from build123d import *

# Parameters (mm, degrees)
BOSS_EXTRUDE1_DEPTH = 25


with BuildPart() as part:
    # Sketch1 → Revolve1 (revolve)
    with BuildSketch(Plane(origin=(0, 0, 0), x_dir=(1, 0, 0), z_dir=(0, 1, 0))):
        Polygon((-85, 0), (-85, 100), (-30, 100), (-30, 433.75), (-65, 433.75), (-65, 478.75), (-45, 478.75), (-17.679491924, 471.429491924), (0, 453.75), (0, 0), align=None)
    revolve(axis=Axis((0, 0, 0), (-1, 0, 0)))

    # Sketch2 → Boss-Extrude1 (add)
    with BuildSketch(Plane.ZY.offset(30)):
        with BuildLine():
            Line((20, 105.830052443), (20, 422.686719096))
            ThreePointArc((20, 422.686719096), (23.183829742, 430.003810253), (30.707964602, 432.661626921))
            ThreePointArc((30.707964602, 432.661626921), (-31.38909354, 432.612745197), (-92.842809365, 423.697150391))
            ThreePointArc((-92.842809365, 423.697150391), (-42.387293117, 411.834770603), (-20, 365.087746302))
            Line((-20, 365.087746302), (-20, 105.830052443))
            ThreePointArc((-20, 105.830052443), (-22.022759648, 99.799825551), (-27.272727273, 96.209138584))
            ThreePointArc((-27.272727273, 96.209138584), (0, 100), (27.272727273, 96.209138584))
            ThreePointArc((27.272727273, 96.209138584), (22.022759648, 99.799825551), (20, 105.830052443))
        make_face()
        with BuildLine():
            Line((83.347135305, 68.214771395), (287.018674676, 310.94106015))
            ThreePointArc((287.018674676, 310.94106015), (294.160965293, 314.499750862), (301.633198614, 311.699335889))
            ThreePointArc((301.633198614, 311.699335889), (254.032671724, 351.577109888), (201.225560333, 384.24905513))
            ThreePointArc((201.225560333, 384.24905513), (232.25173743, 342.729764327), (219.352990909, 292.529191499))
            Line((219.352990909, 292.529191499), (52.70535758, 93.926275782))
            ThreePointArc((52.70535758, 93.926275782), (47.279678663, 90.60705882), (40.949921045, 91.231047163))
            ThreePointArc((40.949921045, 91.231047163), (64.278760969, 76.604444312), (82.734163396, 56.169904816))
            ThreePointArc((82.734163396, 56.169904816), (81.020503963, 62.295144755), (83.347135305, 68.214771395))
        make_face()
        with BuildLine():
            Line((107.6952197, -1.318959311), (419.738121614, 53.702623435))
            ThreePointArc((419.738121614, 53.702623435), (427.496915948, 51.837762766), (431.420906716, 44.889461442))
            ThreePointArc((431.420906716, 44.889461442), (420.58972663, 106.034637518), (401.138253978, 165.006556522))
            ThreePointArc((401.138253978, 165.006556522), (398.217598843, 113.257692306), (356.068279535, 83.092976894))
            Line((356.068279535, 83.092976894), (100.749292594, 38.073350809))
            ThreePointArc((100.749292594, 38.073350809), (94.459429872, 39.018242282), (90.011646197, 43.564934854))
            ThreePointArc((90.011646197, 43.564934854), (98.480775301, 17.364817767), (99.483364979, -10.151851674))
            ThreePointArc((99.483364979, -10.151851674), (102.107854032, -4.358126605), (107.6952197, -1.318959311))
        make_face()
        with BuildLine():
            Line((81.651513899, -70.235534297), (356.057436579, -228.663867624))
            ThreePointArc((356.057436579, -228.663867624), (360.802308533, -235.07969064), (359.341977855, -242.924690904))
            ThreePointArc((359.341977855, -242.924690904), (390.348174112, -189.122620191), (413.353900432, -131.444343727))
            ThreePointArc((413.353900432, -131.444343727), (377.853020062, -169.208912664), (326.175262908, -165.223365075))
            Line((326.175262908, -165.223365075), (101.651513899, -35.594518146))
            ThreePointArc((101.651513899, -35.594518146), (97.440564044, -30.827643459), (96.955921726, -24.485694643))
            ThreePointArc((96.955921726, -24.485694643), (86.602540378, -50), (69.683194454, -71.723443941))
            ThreePointArc((69.683194454, -71.723443941), (75.417804397, -68.972182092), (81.651513899, -70.235534297))
        make_face()
        with BuildLine():
            Line((17.402157289, -106.288122204), (125.773519831, -404.035993705))
            ThreePointArc((125.773519831, -404.035993705), (125.284291084, -412.000744176), (119.122943915, -417.071680569))
            ThreePointArc((119.122943915, -417.071680569), (177.45837269, -395.787302048), (232.156662956, -366.390974705))
            ThreePointArc((232.156662956, -366.390974705), (180.686813825, -372.500786851), (143.661215732, -336.229858273))
            Line((143.661215732, -336.229858273), (54.98986212, -92.607316471))
            ThreePointArc((54.98986212, -92.607316471), (54.828175369, -86.248932215), (58.533443935, -81.079195489))
            ThreePointArc((58.533443935, -81.079195489), (34.202014333, -93.969262079), (7.277482801, -99.73483967))
            ThreePointArc((7.277482801, -99.73483967), (13.438925908, -101.313387037), (17.402157289, -106.288122204))
        make_face()
        with BuildLine():
            Line((-54.98986212, -92.607316471), (-163.361224663, -390.355187972))
            ThreePointArc((-163.361224663, -390.355187972), (-168.855638543, -396.142070634), (-176.835039387, -396.066195661))
            ThreePointArc((-176.835039387, -396.066195661), (-118.466173544, -417.258706591), (-57.66925725, -429.899196636))
            ThreePointArc((-57.66925725, -429.899196636), (-101.024760711, -401.495402985), (-106.073510901, -349.910664006))
            Line((-106.073510901, -349.910664006), (-17.402157289, -106.288122204))
            ThreePointArc((-17.402157289, -106.288122204), (-13.438925908, -101.313387037), (-7.277482801, -99.73483967))
            ThreePointArc((-7.277482801, -99.73483967), (-34.202014333, -93.969262079), (-58.533443935, -81.079195489))
            ThreePointArc((-58.533443935, -81.079195489), (-54.828175369, -86.248932215), (-54.98986212, -92.607316471))
        make_face()
        with BuildLine():
            Line((-101.651513899, -35.594518146), (-376.057436579, -194.022851472))
            ThreePointArc((-376.057436579, -194.022851472), (-383.986138274, -194.924119613), (-390.049942457, -189.736936017))
            ThreePointArc((-390.049942457, -189.736936017), (-358.959080571, -243.490125006), (-320.511091067, -292.252806664))
            ThreePointArc((-320.511091067, -292.252806664), (-335.465726945, -242.625857938), (-306.175262908, -199.864381227))
            Line((-306.175262908, -199.864381227), (-81.651513899, -70.235534297))
            ThreePointArc((-81.651513899, -70.235534297), (-75.417804397, -68.972182092), (-69.683194454, -71.723443941))
            ThreePointArc((-69.683194454, -71.723443941), (-86.602540378, -50), (-96.955921726, -24.485694643))
            ThreePointArc((-96.955921726, -24.485694643), (-97.440564044, -30.827643459), (-101.651513899, -35.594518146))
        make_face()
        with BuildLine():
            Line((-100.749292594, 38.073350809), (-412.792194508, 93.094933555))
            ThreePointArc((-412.792194508, 93.094933555), (-419.445256376, 97.500993314), (-420.75614253, 105.37234468))
            ThreePointArc((-420.75614253, 105.37234468), (-431.491044414, 44.21019216), (-433.38222329, -17.858080426))
            ThreePointArc((-433.38222329, -17.858080426), (-412.938551255, 29.771022524), (-363.014206641, 43.700666774))
            Line((-363.014206641, 43.700666774), (-107.6952197, -1.318959311))
            ThreePointArc((-107.6952197, -1.318959311), (-102.107854032, -4.358126605), (-99.483364979, -10.151851674))
            ThreePointArc((-99.483364979, -10.151851674), (-98.480775301, 17.364817767), (-90.011646197, 43.564934854))
            ThreePointArc((-90.011646197, 43.564934854), (-94.459429872, 39.018242282), (-100.749292594, 38.073350809))
        make_face()
        with BuildLine():
            Line((-52.70535758, 93.926275782), (-256.376896951, 336.652564537))
            ThreePointArc((-256.376896951, 336.652564537), (-258.641277405, 344.304307868), (-254.585867329, 351.176734218))
            ThreePointArc((-254.585867329, 351.176734218), (-302.123553086, 311.224069073), (-343.468996728, 264.892640114))
            ThreePointArc((-343.468996728, 264.892640114), (-297.192838133, 288.237710679), (-249.994768634, 266.817687112))
            Line((-249.994768634, 266.817687112), (-83.347135305, 68.214771395))
            ThreePointArc((-83.347135305, 68.214771395), (-81.020503963, 62.295144755), (-82.734163396, 56.169904816))
            ThreePointArc((-82.734163396, 56.169904816), (-64.278760969, 76.604444312), (-40.949921045, 91.231047163))
            ThreePointArc((-40.949921045, 91.231047163), (-47.279678663, 90.60705882), (-52.70535758, 93.926275782))
        make_face()
    extrude(amount=BOSS_EXTRUDE1_DEPTH)


solid = part.part
Verification items for the finished model (mm, model axes). Give positions to 0.01 mm unless a question says otherwise; leave off trailing zeros. Use one line per item in the form item = value. Start each with the question number.
Q1. Go/stop test with flat-tipped pins: pin 1 Ø1.5 at (x, z) = (-38.5, -259.5) entering from -Y; pin 2 Ø1.5 at (y, z) = (-60, -276.5) entering from -X; pin 3 Ø20 at (x, y) = (-44, 325) entering from +Z; pin 4 Ø6 at (y, z) = (143.5, -254.5) entering from +X. Record where each tip stops, or that it passes through.
Q2. Scan lines: line 1 along Z through (x, y) = (-47, -76); line 2 along Y through (x, z) = (-53, 0); line 3 along Y through (x, z) = (-54.5, -381.5). Record each from-to range of solid material in increasing order. Write a range as [from, to].
Q3. Mould release check, pull along Z, two halves, no side actions. Record for faces 1 (the flat face through (-85, -1, -1)), 2 (the flat face through (-42.3, 65.2, -254.6)): +Z half, -Z half, draft (parallel to the pull), parting line (faces both ways), or undercut.
Evaluation:
q1.pin_1 = -400.79
q1.pin_2 = -30
q1.pin_3 = 360.48
q1.pin_4 = 0
q2.line_1 = [-472.68, -427.04], [-171.64, -91.64], [-64.99, 64.99], [91.64, 171.64], [427.04, 472.68]
q2.line_2 = [-478.75, -433.75], [-100, 478.75]
q2.line_3 = [-289.24, -195.35], [44.07, 87.58], [206.39, 289.24]
q3.face_1 = draft
q3.face_2 = undercut
